Design review of the part built by this model. Coordinates are the model's own, in mm. Round coordinates to 2 decimals unless told otherwise and drop trailing zeros. Write each loop counter-clockwise with the first axis right and the second up, starting at its lowest first coordinate (ties: lowest second). Pieces come first, ordered by that corner, then holes. Notation, with made-up numbers: M 16,81 L 38,81 A20 cw 38,116 Z; hole C 28.5,-15 d5. An arc over 180 degrees is marked long. Use CSV: the item, a comma, the result in double quotes.
Autodesk Inventor part; units mm, degrees
ref_plane "YZ Plane" through (0, 0, 0) normal (1, 0, 0) x (0, 1, 0)
ref_plane "XZ Plane" through (0, 0, 0) normal (0, 1, 0) x (-1, 0, 0)
ref_plane "XY Plane" through (0, 0, 0) normal (0, 0, 1) x (1, 0, 0)
sketch "Skizze1" plane through (0, 0, 0) normal (0, 1, 0) x (-1, 0, 0)
  line L0 (0, 0) -> (180, 0)
  line L1 (180, 0) -> (180, -190)
  line L2 (180, -190) -> (0, -190)
  line L3 (0, -190) -> (0, 0)
  circle A0 centre (165.1, -18.17) radius 2
  circle A1 centre (165.1, -175.65) radius 2
  circle A2 centre (33.02, -175.65) radius 2
  circle A3 centre (10.16, -18.17) radius 2
  dimension "d0" = 190
  dimension "d1" = 180
extrude "Extrusion1" add sketch "Skizze1" along normal blind 4
sketch "Skizze2" plane through (0, 4, 0) normal (0, 1, 0) x (1, 0, 0)
  circle A0 centre (-90, 95) radius 95 construction
  line L0 (0, 190) -> (-180, 190)
  line L1 (-180, 0) -> (0, 0)
  circle A1 centre (-90, 95) radius 4 construction
  circle A2 centre (-90, 107.5) radius 4 construction
  circle A3 centre (-90, 120) radius 4
  circle A4 centre (-90, 132.5) radius 4
  circle A5 centre (-90, 145) radius 4
  line L2 (-180, 190) -> (-180, 0)
  line L3 (-180, 95) -> (0, 95) construction
  line L4 (0, 0) -> (0, 190)
  line L5 (-90, 145) -> (-90, 132.5) construction
  line L6 (-90, 132.5) -> (-90, 120) construction
  line L7 (-90, 120) -> (-90, 107.5) construction
  line L8 (-90, 107.5) -> (-90, 95) construction
  circle A6 centre (-104.7378, 142.7786) radius 4
  circle A7 centre (-118.166, 136.3119) radius 4
  circle A8 centre (-129.0916, 126.1745) radius 4
  circle A9 centre (-136.5437, 113.2671) radius 4
  circle A10 centre (-139.8602, 98.7365) radius 4
  circle A11 centre (-138.7464, 83.874) radius 4
  circle A12 centre (-133.3013, 70) radius 4
  circle A13 centre (-124.0086, 58.3474) radius 4
  circle A14 centre (-111.6942, 49.9516) radius 4
  circle A15 centre (-97.4521, 45.5585) radius 4
  circle A16 centre (-82.5479, 45.5585) radius 4
  circle A17 centre (-68.3058, 49.9516) radius 4
  circle A18 centre (-55.9914, 58.3474) radius 4
  circle A19 centre (-46.6987, 70) radius 4
  circle A20 centre (-41.2536, 83.874) radius 4
  circle A21 centre (-40.1398, 98.7365) radius 4
  circle A22 centre (-43.4563, 113.2671) radius 4
  circle A23 centre (-50.9084, 126.1745) radius 4
  circle A24 centre (-61.834, 136.3119) radius 4
  circle A25 centre (-106.2706, 128.7863) radius 4
  circle A26 centre (-119.3187, 118.3809) radius 4
  circle A27 centre (-126.5598, 103.3445) radius 4
  circle A28 centre (-126.5598, 86.6555) radius 4
  circle A29 centre (-119.3187, 71.6191) radius 4
  circle A30 centre (-106.2706, 61.2137) radius 4
  circle A31 centre (-90, 57.5) radius 4
  circle A32 centre (-73.7294, 61.2137) radius 4
  circle A33 centre (-60.6813, 71.6191) radius 4
  circle A34 centre (-53.4402, 86.6555) radius 4
  circle A35 centre (-53.4402, 103.3445) radius 4
  circle A36 centre (-60.6813, 118.3809) radius 4
  circle A37 centre (-73.7294, 128.7863) radius 4
  circle A38 centre (-109.5458, 110.5872) radius 4
  circle A39 centre (-114.3732, 89.437) radius 4
  circle A40 centre (-100.8471, 72.4758) radius 4
  circle A41 centre (-79.1529, 72.4758) radius 4
  circle A42 centre (-65.6268, 89.437) radius 4
  circle A43 centre (-70.4542, 110.5872) radius 4
  circle A44 centre (-75.2622, 142.7786) radius 4
  circle A45 centre (-37.5, 147.5) radius 2
  circle A46 centre (-37.5, 42.5) radius 2
  circle A47 centre (-142.5, 42.5) radius 2
  circle A48 centre (-142.5, 147.5) radius 2
  line L9 (-142.5, 147.5) -> (-37.5, 147.5) construction
  line L10 (-37.5, 147.5) -> (-37.5, 42.5) construction
  line L11 (-37.5, 42.5) -> (-142.5, 42.5) construction
  line L12 (-142.5, 42.5) -> (-142.5, 147.5) construction
  line L13 (-90, 147.5) -> (-90, 95) construction
  line L14 (-90, 95) -> (-37.5, 95) construction
  dimension "d4" = 8
  dimension "d5" = 50
  dimension "d8" = 360
  dimension "d12" = 360
  dimension "d16" = 360
  dimension "d20" = 4
  dimension "d21" = 105
extrude "Extrusion2" cut sketch "Skizze2" against normal blind 4 contours A3 | A4 | A5 | A6 | A7 | A8 | A9 | A10 | A11 | A12 | A13 | A14 | A15 | A16 | A17 | A18 | A19 | A20 | A21 | A22 | A23 | A24 | A25 | A26 | A27 | A28 | A29 | A30 | A31 | A32 | A33 | A34 | A35 | A36 | A37 | A38 | A39 | A40 | A41 | A42 | A43 | A44 | A45 | A46 | A47 | A48
sketch "Skizze3" plane through (0, 0, 0) normal (0, -1, 0) x (1, 0, 0)
  line L0 (0, -190) -> (-180, -190)
  line L1 (-180, -190) -> (-138, -190)
  line L2 (-138, -190) -> (-138, -200)
  line L3 (-138, -200) -> (-180, -200)
  line L4 (-180, -200) -> (-180, -190)
  line L5 (-180, 0) -> (-138, 0)
  line L6 (-138, 0) -> (-138, 10)
  line L7 (-138, 10) -> (-180, 10)
  line L8 (-180, 10) -> (-180, 0)
  line L9 (0, 0) -> (0, -190)
  dimension "d22" = 10
  dimension "d23" = 138
extrude "Extrusion3" add sketch "Skizze3" against normal blind 4
properties part number "Platte2" material "Pappel"
1) Add section A-A on x = -26.5. Write out the cut boundary in (y, z), then the cut area to 3 significant figures.
Answers:
outline,"M 0,-190 L 4,-190 L 4,0 L 0,0 Z"
area,"760 mm²"
2) For pin 1 Ø7 at (x, z) = (-55.99, -58.35) entering from +Y, flat-tipped, find the tip position at first contact; note if it passes through.
Answers:
pin 1,"through"
3) Wall thickness on line 1 along X through (y, z) = (2.5, -103.5); line 2 along X through (y, z) = (0.5, -104); line 3 along X through (y, z) = (1.25, -144.5): over which ranges is each line inside the solid? List them lowest first. Write a range as [from, to].
Answers:
line 1,"[-180, -130.56], [-122.56, -57.44], [-49.44, 0]"
line 2,"[-180, -130.51], [-122.61, -57.39], [-49.49, 0]"
line 3,"[-180, -108.35], [-101.13, -93.97], [-86.03, -78.87], [-71.65, 0]"
4) Add section B-B on y = 0.8. Give the number of separate pieces and of enclosed holes in the cut face, then the cut area to 3 significant figures.
Answers:
separate pieces,"1"
enclosed holes,"50"
area,"32,800 mm²"
5) The part is to be moulded in two halves that separate along Z. For faces 1 (the face through (-89, 4, -94)), 2 (the face through (-119, 2, -132.4)), say which applies: released by +Z, released by -Z, zero draft, split by the parting line, or undercut.
Answers:
face 1,"zero draft"
face 2,"undercut"
